Could you check a few things on this drawing? It's one solid part, dimensions in mm from its lowest x, y, z. A direction names the side the tool comes from. Coordinates: 2 decimals unless noted, no trailing zeros. Write each loop counter-clockwise with the first axis right and the second up, starting at its lowest first coordinate (ties: lowest second). Pieces come first, ordered by that corner, then holes. Notation, with made-up numbers: (78, 80.25) - (124, 80.25) arc R3 cw to (124, 85.25) - close; hole circle Ø2 at (-1, 56.25). An arc over 180 degrees is marked (long way). Use one line per item in the form item = value. Start each with the question number.
(1) For pin 1 Ø7.5 at (x, z) = (15.5, 3.5) entering from -Y; pin 2 Ø4 at (y, z) = (6, 4.5) entering from +X (1 decimal); pin 3 Ø1.5 at (x, y) = (125, 80) entering from -Z; pin 4 Ø4 at (y, z) = (6, 6.5) entering from -X (1 decimal), each with a flat end and sliding along its axis, tell me the tip position at first contact or that it passes through.
(2) On a 3-axis mill with a long thin cutter (end or side, diameter ignored), from which of +Z, -Z, +X, -X, +Y, -Y can I reach the whole of each face in a straight line? I mean the marked faces 4, 5, 6 and 7. Say none if no direction works.
(3) If we section it at A-A on x = 120.65: Please give me the cut outline in (y, z), then the cut area to 3 significant figures.
(4) If I drill on probe 1 along Y at (x, z) = (120.65, 7.5); probe 2 along X at (y, z) = (10.5, 7.75) (1 decimal); probe 3 along Y at (x, z) = (96, 10.75), over which ranges is the centre line in solid material (lowest first)? Write a range as from..to.
(5) If we section it at B-B on y = 66.04: Please give me the cut outline in (x, z).
(6) Thinking about a two-plate mould opening in X: for the marked faces 1, 2 and 3, which applies, pulls with the +X half, pulls with the -X half, needs draft (parallel to the pull), parting line crosses it, or undercut?
(7) If we section it at D-D on y = 84.5: Please give me the cut outline in (x, z), then the cut area to 3 significant figures.
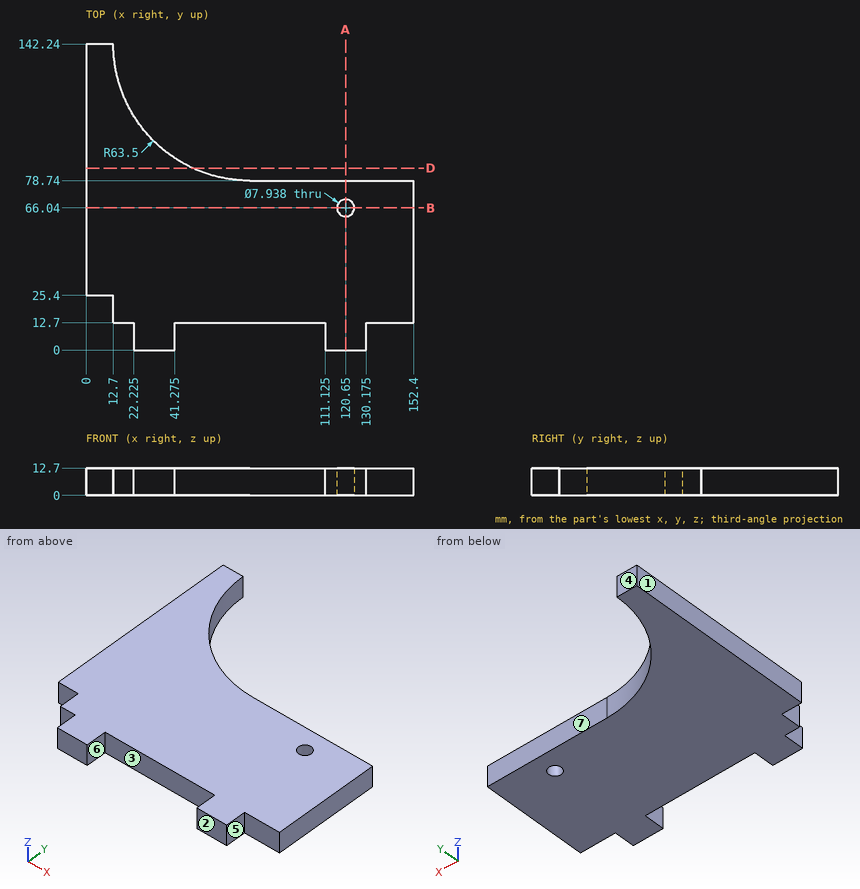
Reported:
q1.pin_1 = 12.7
q1.pin_2 = 130.2
q1.pin_3 = through
q1.pin_4 = 22.2
q2.face_4 = +Z, -Z, +X, -X, +Y
q2.face_5 = +Z, -Z, +X, -Y
q2.face_6 = +Z, -Z, -Y
q2.face_7 = +Z, -Z, +X, +Y
q3.outline = (0, 0) - (62.07, 0) - (62.07, 12.7) - (0, 12.7) - close; (70.01, 0) - (78.74, 0) - (78.74, 12.7) - (70.01, 12.7) - close
q3.area = 899 mm2
q4.probe_1 = 0..62.07, 70.01..78.74
q4.probe_2 = 22.2..41.3, 111.1..130.2
q4.probe_3 = 12.7..78.74
q5.outline = (0, 0) - (116.68, 0) - (116.68, 12.7) - (0, 12.7) - close; (124.62, 0) - (152.4, 0) - (152.4, 12.7) - (124.62, 12.7) - close
q6.face_1 = pulls with the -X half
q6.face_2 = needs draft
q6.face_3 = undercut
q7.outline = (0, 0) - (49.77, 0) - (49.77, 12.7) - (0, 12.7) - close
q7.area = 632 mm2
